Here's the drawing with two shaded views (mm, measured from the low corner). I have some questions. Give positions to 0.01 mm unless a question says otherwise; leave off trailing zeros. Order: outer loops, then holes, each group sorted by start corner. A loop starts at its lowest first (then second) coordinate and runs counter-clockwise, first axis right, second up. Notation, with made-up numbers: (57, 73.25) - (112, 73.25) arc R33 cw to (112, 105.25) - close; hole circle Ø4 at (1.25, -24.5). An arc over 180 degrees is marked (long way). Use one line per item in the form item = value. Start each with the question number.
1) Suppose I cut it at A-A, the plane x = 272.5. Write out the boundary of the cut face in (y, z), and give its area (3 significant figures).
2) Suppose I cut it at B-B, the plane y = 49. Write out the boundary of the cut face in (x, z), and give its area (3 significant figures).
3) Suppose I cut it at D-D, the plane z = 30. Write out the boundary of the cut face in (x, y).
4) For pin 1 (20 mm diameter, centred on y = 22.5, z = 308.5, fed in from +X), with a flat end and sliding along its axis, tell me the tip position at first contact or that it passes through.
5) Please list where these lines run through material, in increasing order: probe 1 along Z at (x, y) = (201, 432); probe 2 along X at (y, z) = (62, 25).
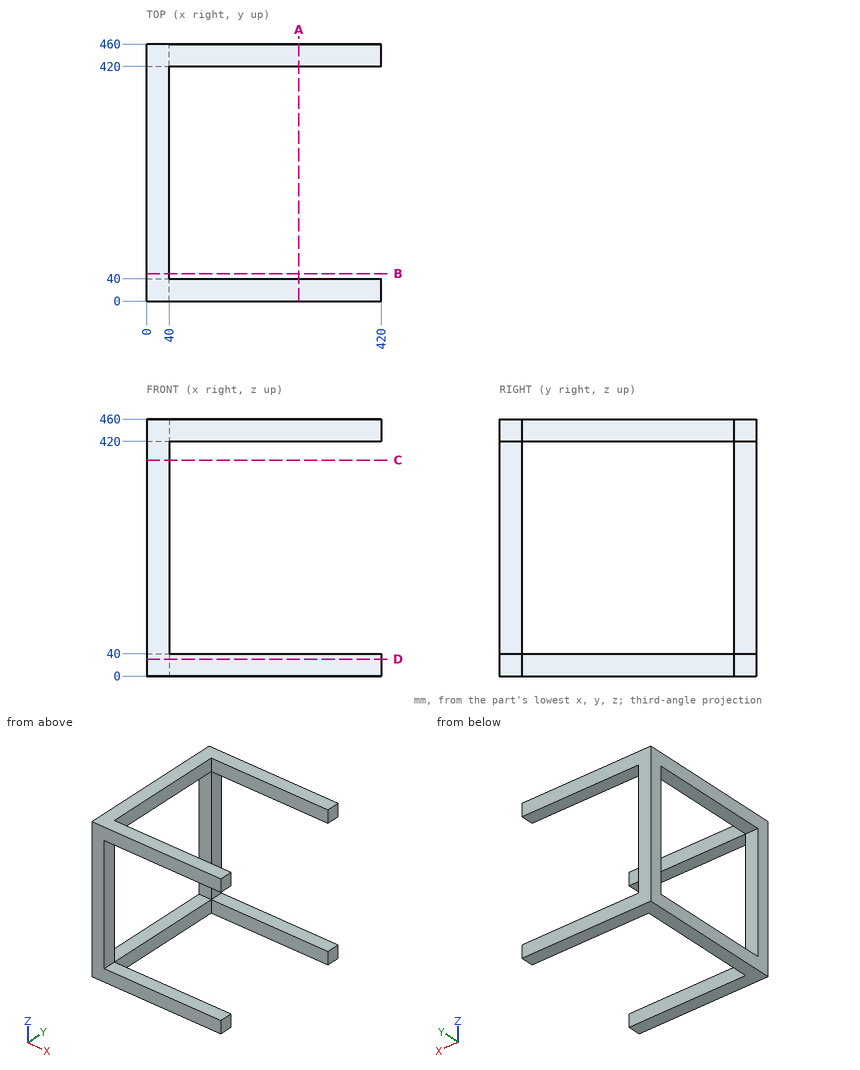
Result sheet:
q1.outline = (0, 0) - (40, 0) - (40, 40) - (0, 40) - close; (0, 420) - (40, 420) - (40, 460) - (0, 460) - close; (420, 0) - (460, 0) - (460, 40) - (420, 40) - close; (420, 420) - (460, 420) - (460, 460) - (420, 460) - close
q1.area = 6,400 mm²
q2.outline = (0, 0) - (40, 0) - (40, 40) - (0, 40) - close; (0, 420) - (40, 420) - (40, 460) - (0, 460) - close
q2.area = 3,200 mm²
q3.outline = (0, 0) - (420, 0) - (420, 40) - (40, 40) - (40, 420) - (420, 420) - (420, 460) - (0, 460) - close
q4.pin_1 = 40
q5.probe_1 = 0 to 40, 420 to 460
q5.probe_2 = 0 to 40
